from build123d import *

# Parameters (mm, degrees)
SKETCH1_R           = 5
BOSS_EXTRUDE1_DEPTH = 5
SKETCH3_R           = 4
CUT_EXTRUDE1_DEPTH  = 4.5
SKETCH4_R           = 0.3
CUT_EXTRUDE2_DEPTH  = 9.381527307


with BuildPart() as part:
    # Sketch1 → Boss-Extrude1 (new body)
    with BuildSketch(Plane.XY):
        Circle(SKETCH1_R)
    extrude(amount=BOSS_EXTRUDE1_DEPTH)

    # Sketch3 → Cut-Extrude1 (cut)
    with BuildSketch(Plane.XY.offset(5)):
        Circle(SKETCH3_R)
    extrude(amount=-CUT_EXTRUDE1_DEPTH, mode=Mode.SUBTRACT)

    # Sketch4 → Cut-Extrude2 (cut, through all)
    with BuildSketch(Plane.XY.offset(0.5)):
        with Locations((1.29, 0)):
            Circle(SKETCH4_R)
        with Locations((-1.29, 0)):
            Circle(SKETCH4_R)
    extrude(amount=-CUT_EXTRUDE2_DEPTH, mode=Mode.SUBTRACT)


solid = part.part
For this review, take the finished solid that the model builds, in its own axes (mm). Round coordinates to 2 decimals unless told otherwise and drop trailing zeros. Loops run counter-clockwise (first coordinate to the right, second up) from the corner with the lowest first, then second, coordinate; pieces in that order, holes last. Notation, with made-up numbers: (27, 72.25) - (59, 72.25) arc R7 ccw to (59, 80.25) - close; hole circle Ø11 at (51.25, -9). An arc over 180 degrees is marked (long way). Put each result on its own line as item: value. Start each with the question number.
1. Consider section A-A on y = 0. State the section outline as (x, z) points, plus the area to 3 significant figures.
2. For probe 1 along Z at (x, y) = (-3, 2); probe 2 along Y at (x, z) = (-3, 0.35); probe 3 along X at (y, z) = (-1, 3.85), list the stretches that pass through material, from the lowest coordinate up. Write a range as [from, to].
3. Consider section C-C on z = 1.8. State the section outline as (x, y) points.
4. Consider section B-B on x = 0. State the section outline as (y, z) points.
5. Mouldability with a two-part tool opening along X and no side actions: class faces 1 (the cylindrical face through (-0.867, -3.905, 2.782)), 2 (the flat face through (0, 0, 0)), 3 (the cylindrical face through (-1.08, -4.88, 2.46)) as +X half, -X half, draft (parallel to the pull), parting line (faces both ways), or undercut.
6. Consider section D-D on y = 3. State the section outline as (x, z) points, plus the area to 3 significant figures.
7. Insertion check: P1, Ø1, axis at y = 3, z = 1, coming from the -X side; P2, Ø6, axis at x = -1.5, y = -0.5, coming from the +Z side; P3, Ø2, axis at y = 2.5, z = 0.5, coming from the -X side; P4, Ø2, axis at x = -2.5, z = 1, coming from the +Y side. Each pin has a flat end and moves straight along its axis. Give the tip position at first contact, or say it passes through.
Result sheet:
1. outline: (-5, 0) - (-1.59, 0) - (-1.59, 0.5) - (-4, 0.5) - (-4, 5) - (-5, 5) - close; (-0.99, 0) - (0.99, 0) - (0.99, 0.5) - (-0.99, 0.5) - close; (1.59, 0) - (5, 0) - (5, 5) - (4, 5) - (4, 0.5) - (1.59, 0.5) - close
1. area: 13.4 mm^2
2. probe 1: [0, 0.5]
2. probe 2: [-4, 4]
2. probe 3: [-4.9, -3.87], [3.87, 4.9]
3. outline: circle Ø10 at (0, 0); hole circle Ø8 at (0, 0)
4. outline: (-5, 0) - (5, 0) - (5, 5) - (4, 5) - (4, 0.5) - (-4, 0.5) - (-4, 5) - (-5, 5) - close
5. face 1: undercut
5. face 2: draft
5. face 3: parting line
6. outline: (-4, 0) - (4, 0) - (4, 5) - (2.65, 5) - (2.65, 0.5) - (-2.65, 0.5) - (-2.65, 5) - (-4, 5) - close
6. area: 16.2 mm^2
7. P1: x = -4.33
7. P2: z = 5
7. P3: x = -4.77
7. P4: y = 4.77
